Geometry check sheet. Reference: the model listing, model coordinates, mm. A direction names the side the tool comes from. Coordinates: 2 decimals unless noted, no trailing zeros. Loops run counter-clockwise (first coordinate to the right, second up) from the corner with the lowest first, then second, coordinate; pieces in that order, holes last. Notation, with made-up numbers: M 60.5,-12.5 L 114.5,-12.5 A14 ccw 114.5,4.5 Z; hole C 49,73.5 d11. An arc over 180 degrees is marked long. Use CSV: the item, a comma, the result in double quotes.
```python
from build123d import *

# Parameters (mm, degrees)
SKETCH3_R           = 17.78
SKETCH3_R_2         = 15.24
BOSS_EXTRUDE1_DEPTH = 177.8


with BuildPart() as part:
    # Sketch2 → Loft1 section 0
    with BuildSketch(Plane(origin=(0, 50.8, 0), x_dir=(1, 0, 0), z_dir=(0, 1, 0))):
        with BuildLine():
            Line((-25.4, -25.4), (25.4, -25.4))
            Line((25.4, -25.4), (25.4, 25.4))
            Line((25.4, 25.4), (-25.4, 25.4))
            Line((-25.4, 25.4), (-25.4, -25.4))
        make_face()
    # Sketch1 → Loft1 section 1
    with BuildSketch(Plane(origin=(0, 0, 0), x_dir=(1, 0, 0), z_dir=(0, 1, 0))):
        with BuildLine():
            Line((-63.5, -63.5), (63.5, -63.5))
            Line((63.5, -63.5), (63.5, 63.5))
            Line((63.5, 63.5), (-63.5, 63.5))
            Line((-63.5, 63.5), (-63.5, -63.5))
        make_face()
    loft()

    # Sketch3 → Boss-Extrude1 (add)
    with BuildSketch(Plane(origin=(0, 50.8, 0), x_dir=(1, 0, 0), z_dir=(0, 1, 0))):
        with Locations(Location((0, 0, 0), (0, 0, 90))):
            Circle(SKETCH3_R)
        with Locations(Location((0, 0, 0), (0, 0, 270))):
            Circle(SKETCH3_R_2, mode=Mode.SUBTRACT)
    extrude(amount=BOSS_EXTRUDE1_DEPTH)


solid = part.part
```
1. Thickness scan on line 1 (X direction, y = 192, z = 0); line 2 (Y direction, x = -25, z = 14); line 3 (Y direction, x = 35.5, z = -56). Record the ranges inside material, lowest first. Write a range as [from, to].
The answers:
line 1,"[-17.78, -15.24], [15.24, 17.78]"
line 2,"[0, 50.8]"
line 3,"[0, 10]"
2. Gauge pin test, flat ends, axial feed: P1, Ø15, axis at x = 0, z = 6.5, coming from the +Y side; P2, Ø5, axis at x = -18.5, z = 38.5, coming from the +Y side; P3, Ø5, axis at x = -42.5, z = 30.5, coming from the +Y side. Record the tip position at first contact, or that the pin passes through.
The answers:
P1,"y = 50.8"
P2,"y = 36.67"
P3,"y = 31.33"
3. Set-up check for faces 4 (the flat face through (-13.3, 228.6, 8)), 5 (the cylindrical face through (15.11, 138.46, -1.98)): record each of +Z, -Z, +X, -X, +Y, -Y from which the full face is reachable in a straight line by a thin tool's end or side.
The answers:
face 4,"+Z, -Z, +X, -X, +Y"
face 5,"+Y"
4. Section check A-A, the plane y = 61.5. Record the cut outline in (x, z), plus the area to 3 significant figures.
The answers:
outline,"C 0,0 d35.56; hole C 0,0 d30.48"
area,"263 mm^2"
5. Release check for a two-part mould opening along X. For faces 1 (the flat face through (0, 50.8, 0)), 2 (the cylindrical face through (17.36, 138.46, 3.85)), 3 (the flat face through (-13, 50.8, -13)) record: +X half, -X half, draft (parallel to the pull), parting line (faces both ways), or undercut.
The answers:
face 1,"undercut"
face 2,"parting line"
face 3,"draft"
